from build123d import *

# Parameters (mm, degrees)
SKETCH1_W          = 2.794
SKETCH1_H          = 10.0838
SKETCH7_W          = 10.16
SKETCH7_H          = 7.5438
CUT_REVOLVE2_ANGLE = 20
SKETCH8_W          = 10.16
SKETCH8_H          = 5.08
CUT_REVOLVE3_ANGLE = 10
SKETCH9_W          = 10.16
SKETCH9_H          = 2.54
CUT_REVOLVE4_ANGLE = 5
CIRPATTERN2_COUNT  = 2
FILLET1_R          = 2.54
FILLET2_R          = 1.27


with BuildPart() as part:
    # Sketch1 → Revolve1 (revolve)
    with BuildSketch(Plane.XY, mode=Mode.PRIVATE) as revolve1_sk:
        with Locations((-19.177, 0)):
            Rectangle(SKETCH1_W, SKETCH1_H)
    revolve(revolve1_sk.sketch.rotate(Axis((0, 0, 0), (0, 1, 0)), 270), axis=Axis((0, 0, 0), (0, 1, 0)))

    # Sketch2 → Cut-Revolve1 (revolve, cut)
    with BuildSketch(Plane.XY, mode=Mode.PRIVATE) as cut_revolve1_sk:
        with BuildLine():
            Line((-17.78, 3.7719), (-15.24, 3.7719))
            Line((-15.24, 3.7719), (-15.24, -3.7719))
            Line((-15.24, -3.7719), (-17.78, -3.7719))
            ThreePointArc((-17.78, -3.7719), (-18.57375, 0), (-17.78, 3.7719))
        make_face()
    revolve(cut_revolve1_sk.sketch.rotate(Axis((0, 0, 0), (0, 1, 0)), 270), axis=Axis((0, 0, 0), (0, 1, 0)), mode=Mode.SUBTRACT)

    # Sketch7 → Cut-Revolve2 (revolve, symmetric, cut)
    with BuildSketch(Plane.XY) as cut_revolve2_sk:
        with Locations((-22.86, 0)):
            Rectangle(SKETCH7_W, SKETCH7_H)
    cut_revolve2 = revolve(axis=Axis((0, 0, 0), (0, 1, 0)), revolution_arc=CUT_REVOLVE2_ANGLE / 2, mode=Mode.SUBTRACT)
    cut_revolve2 = cut_revolve2 + revolve(cut_revolve2_sk.sketch, axis=Axis((0, 0, 0), (0, -1, 0)), revolution_arc=CUT_REVOLVE2_ANGLE / 2, mode=Mode.SUBTRACT)

    # Sketch8 → Cut-Revolve3 (revolve, cut)
    with BuildSketch(Plane(origin=(0, 0, 0), x_dir=(0.9848077530122081, 0, 0.17364817766693072), z_dir=(-0.17364817766693072, 0, 0.9848077530122081))):
        with Locations((-23.302480977, 0)):
            Rectangle(SKETCH8_W, SKETCH8_H)
    cut_revolve3 = revolve(axis=Axis((0, 0, 0), (0, -1, 0)), revolution_arc=CUT_REVOLVE3_ANGLE, mode=Mode.SUBTRACT)

    # Sketch9 → Cut-Revolve4 (revolve, cut)
    with BuildSketch(Plane(origin=(0, 0, 0), x_dir=(-0.9848077530122081, 0, 0.17364817766693075), z_dir=(-0.17364817766693075, 0, -0.9848077530122081))):
        with Locations((23.567180389, 0)):
            Rectangle(SKETCH9_W, SKETCH9_H)
    cut_revolve4 = revolve(axis=Axis((0, 0, 0), (0, 1, 0)), revolution_arc=CUT_REVOLVE4_ANGLE, mode=Mode.SUBTRACT)

    # CirPattern2: Cut-Revolve2, Cut-Revolve3, Cut-Revolve4 ×2 about axis
    cirpattern2_axis = Axis((0, 0, 0), (0, 1, 0))
    add([cut_revolve2.rotate(cirpattern2_axis, i * 360 / CIRPATTERN2_COUNT) for i in range(1, CIRPATTERN2_COUNT)], mode=Mode.SUBTRACT)
    add([cut_revolve3.rotate(cirpattern2_axis, i * 360 / CIRPATTERN2_COUNT) for i in range(1, CIRPATTERN2_COUNT)], mode=Mode.SUBTRACT)
    add([cut_revolve4.rotate(cirpattern2_axis, i * 360 / CIRPATTERN2_COUNT) for i in range(1, CIRPATTERN2_COUNT)], mode=Mode.SUBTRACT)

    # Fillet1
    fillet1_edges = [part.edges().sort_by_distance(p)[0] for p in [
        (18.228383443, 2.54, 6.634588992),
        (18.228383443, -2.54, 6.634588992),
        (-18.228383443, -2.54, -6.634588992),
        (-18.228383443, 2.54, -6.634588992),
    ]]
    fillet(fillet1_edges, radius=FILLET1_R - 0.0001)  # a hair under: the kernel refuses the full size

    # Fillet2
    fillet2_edges = [part.edges().sort_by_distance(p)[0] for p in [
        (-18.865101471, -1.27, 5.054888704),
        (-18.865101471, 1.27, 5.054888704),
        (18.865101471, -1.27, -5.054888704),
        (18.865101471, 1.27, -5.054888704),
    ]]
    fillet(fillet2_edges, radius=FILLET2_R - 0.0001)  # a hair under: the kernel refuses the full size


solid = part.part
Verification items for the finished model (mm, model axes). A direction names the side the tool comes from. Give positions to 0.01 mm unless a question says otherwise; leave off trailing zeros. Write each loop counter-clockwise with the first axis right and the second up, starting at its lowest first coordinate (ties: lowest second). Pieces come first, ordered by that corner, then holes. Notation, with made-up numbers: M 51,14 L 81,14 A29 cw 81,34 Z; hole C 35,15 d4. An arc over 180 degrees is marked long. Put each result on its own line as item: value. Start each with the question number.
1. Section check A-A (z = 0). Record the cut outline in (x, y), and give its area (3 significant figures).
2. Go/stop test with flat-tipped pins: pin 1 Ø1.5 at (y, z) = (1, -13.5) entering from +X; pin 2 Ø5 at (y, z) = (1.5, -1) entering from +X; pin 3 Ø21.5 at (x, z) = (0, 0) entering from -Y; pin 4 Ø2 at (x, y) = (-3, 3) entering from +Z. Record where each tip stops, or that it passes through.
3. Set-up check for faces 5 (the face through (18.253, 0.071, -9.494)), 6 (the face through (-18.905, 3.165, -3.333)), 7 (the face through (19, -2.54, 4)): record each of +Z, -Z, +X, -X, +Y, -Y from which the full face is reachable in a straight line by a thin tool's end or side.
4. Section check B-B (y = 4.25). Record the cut outline in (x, z), and give its area (3 significant figures).
5. Draft check along Y on faces 1 (the face through (19, 3.772, 0)), 2 (the face through (6, 5.042, 17)), 3 (the face through (6, -5.042, 17)), 4 (the face through (-18.64, 1.78, -6.01)). Enter one of: +Y half, -Y half, draft (parallel to the pull), parting line (faces both ways), or undercut.
6. Scan lines: line 1 along X through (y, z) = (-4.65, 0); line 2 along Z through (x, y) = (-3.5, -1.5); line 3 along Z through (x, y) = (8, -2). Record each from-to range of solid material in increasing order. Write a range as [from, to].
Answer list:
1. outline: M -20.57,-5.04 L -17.78,-5.04 L -17.78,-3.77 L -20.57,-3.77 Z; M -20.57,3.77 L -17.78,3.77 L -17.78,5.04 L -20.57,5.04 Z; M 17.78,-5.04 L 20.57,-5.04 L 20.57,-3.77 L 17.78,-3.77 Z; M 17.78,3.77 L 20.57,3.77 L 20.57,5.04 L 17.78,5.04 Z
1. area: 14.2 mm2
2. pin 1: x = 16.15
2. pin 2: x = 20.57
2. pin 3: through
2. pin 4: z = 20.48
3. face 5: +Y, -Y
3. face 6: -X
3. face 7: +X
4. outline: C 0,0 d41.15; hole C 0,0 d35.56
4. area: 337 mm2
5. face 1: undercut
5. face 2: +Y half
5. face 3: -Y half
5. face 4: undercut
6. line 1: [-20.57, -17.78], [17.78, 20.57]
6. line 2: [-20.27, -18.12], [18.12, 20.27]
6. line 3: [-18.95, -16.52], [16.52, 18.95]
